Autodesk Inventor part; units mm, degrees
ref_plane "YZ Plane" through (0, 0, 0) normal (1, 0, 0) x (0, 1, 0)
ref_plane "XZ Plane" through (0, 0, 0) normal (0, 1, 0) x (-1, 0, 0)
ref_plane "XY Plane" through (0, 0, 0) normal (0, 0, 1) x (1, 0, 0)
sketch "Sketch2" plane through (0, 0, 0) normal (0, 0, 1) x (1, 0, 0)
  line L0 (27.4963, -15.875) -> (0, 0) construction
  arc A0 (-38.4948, -9.525) -> (-27.4963, -28.575) centre (-27.4963, -15.875) ccw
  arc A1 (27.4963, -28.575) -> (38.4948, -9.525) centre (27.4963, -15.875) ccw
  arc A2 (10.9985, 38.1) -> (-10.9985, 38.1) centre (0, 31.75) ccw
  line L1 (-38.4948, -9.525) -> (-10.9985, 38.1)
  line L2 (10.9985, 38.1) -> (38.4948, -9.525)
  line L3 (27.4963, -28.575) -> (-27.4963, -28.575)
  point P0 (-25.1827, 3.3154)
  point P1 (-20.1512, -15.4625)
  point P2 (-3.3154, -25.1827)
  point P3 (15.4625, -20.1512)
  point P4 (25.1827, -3.3154)
  point P5 (20.1512, 15.4625)
  point P6 (3.3154, 25.1827)
  point P7 (-15.4625, 20.1512)
  dimension "d74" = 31.75
  dimension "d77" = 360
  dimension "d80" = 25.4
  dimension "d83" = 360
  dimension "d92" = 12.7
extrude "Plate2" add sketch "Sketch2" along normal blind 4.7625
hole "Hole3" at (-27.4963, -15.875, 0) at (0, 31.75, 0) at (27.4963, -15.875, 0) direction (0, 0, 1) diameter 6.5278 end through all
hole "Hole4" at (0, 0, 0) direction (0, 0, 1) diameter 28.575 end through all
hole "Hole5" at (-25.1827, 3.3154, 0) at (15.4625, -20.1512, 0) at (25.1827, -3.3154, 0) at (-15.4625, 20.1512, 0) direction (0, 0, 1) diameter 4.9784 end through all
equation "\"BendRadius\" = Thickness"
equation "\"BendReliefWidth\" = Thickness"
equation "\"BendReliefDepth\" = 0.5 * Thickness"
equation "\"CornerReliefSize\" = 4 * Thickness"
equation "\"MinimumRemnant\" = 2 * Thickness"
equation "\"TransitionRadius\" = BendRadius"
equation "\"JacobiRadiusSize\" = BendRadius"
equation "\"GapSize\" = Thickness"
properties part number "PLATE,TURRET,MOTOR,MOUNT" material "Aluminum 6061"
Geometry check sheet. Reference: the model listing, model coordinates, mm. Round coordinates to 2 decimals unless told otherwise and drop trailing zeros. Order: outer loops, then holes, each group sorted by start corner. A loop starts at its lowest first (then second) coordinate and runs counter-clockwise, first axis right, second up. Notation, with made-up numbers: (54, 84.5) -> (95, 84.5) arc R28 cw to (95, 107.5) -> close; hole circle Ø5 at (-7.75, -34.75). An arc over 180 degrees is marked (long way). Return JSON: item names as keys, results as strings. Group by question number.
Q1. Section check D-D, the plane y = 9.5. Record the boundary of the cut face in (x, z).
Q2. Section check A-A, the plane x = 0. Record the boundary of the cut face in (y, z) (1 decimal).
Q3. Material ranges on probe 1 along Y at (x, z) = (25, 1.4) (3 decimals); probe 2 along Y at (x, z) = (2, 3.4) (3 decimals); probe 3 along X at (y, z) = (-2, 4.3), recorded low to high. Write a range as from..to.
Q4. Gauge pin test, flat ends, axial feed: pin 1 (4.5 mm diameter, centred on x = -25.18, y = 3.32, fed in from -Z); pin 2 (2 mm diameter, centred on x = 28, z = 3.5, fed in from +Y); pin 3 (1.5 mm diameter, centred on y = 35, z = 2.5, fed in from -X). Record the tip position at first contact, or that the pin passes through.
Q5. Section check B-B, the plane y = 31.75. Record the boundary of the cut face in (x, z).
Q6. Release check for a two-part mould opening along X. For faces 1 (the flat face through (-1, -16, 4.762)), 2 (the cylindrical face through (-38.4, -22.39, 2.35)), 3 (the cylindrical face through (38.59, -22.06, 2.35)), 4 (the cylindrical face through (27.61, -3.86, 2.41)) record: released by +X, released by -X, zero draft, split by the parting line, or undercut.
Q7. Section check C-C, the plane z = 1.7. Count the separate pieces of the cut face and the enclosed holes in it, plus the area to 3 significant figures.
Numbers:
{
 "1": {"outline": "(-27.51, 0) -> (-10.67, 0) -> (-10.67, 4.76) -> (-27.51, 4.76) -> close; (10.67, 0) -> (27.51, 0) -> (27.51, 4.76) -> (10.67, 4.76) -> close"},
 "2": {"outline": "(-28.6, 0) -> (-14.3, 0) -> (-14.3, 4.8) -> (-28.6, 4.8) -> close; (14.3, 0) -> (28.5, 0) -> (28.5, 4.8) -> (14.3, 4.8) -> close; (35, 0) -> (44.4, 0) -> (44.4, 4.8) -> (35, 4.8) -> close"},
 "3": {"probe 1": "-28.575..-17.978, -13.772..-5.798, -0.833..13.849", "probe 2": "-28.575..-14.147, 14.147..29.171, 34.329..44.292", "probe 3": "-34.15..-14.15, 14.15..23.07, 27.3..34.15"},
 "4": {"pin 1": "through", "pin 2": "y = 10.38", "pin 3": "x = -13.22"},
 "5": {"outline": "(-14.66, 0) -> (-3.26, 0) -> (-3.26, 4.76) -> (-14.66, 4.76) -> close; (3.26, 0) -> (14.66, 0) -> (14.66, 4.76) -> (3.26, 4.76) -> close"},
 "6": {"face 1": "zero draft", "face 2": "released by -X", "face 3": "released by +X", "face 4": "undercut"},
 "7": {"separate pieces": "1", "enclosed holes": "8", "area": "3,090 mm^2"}
}
